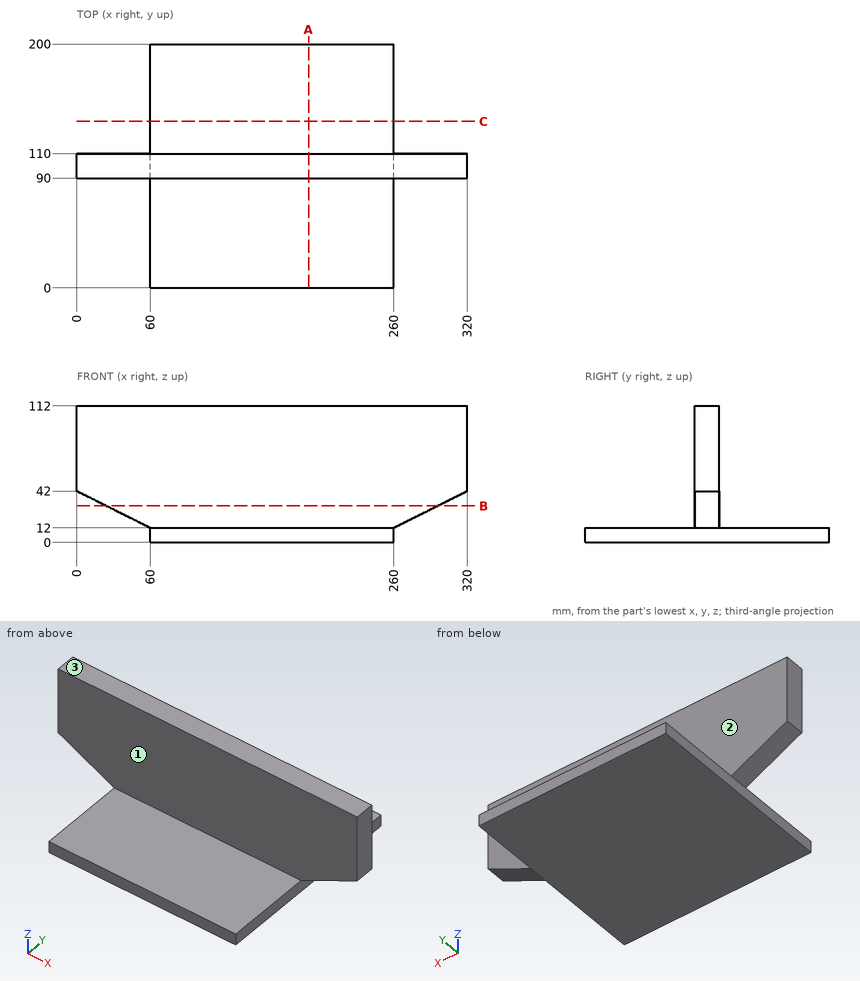
Input: dimensioned drawing with shaded views. Units: mm. Origin: part minimum x, y, z. A direction names the side the tool comes from. Round coordinates to 2 decimals unless told otherwise and drop trailing zeros. Loops run counter-clockwise (first coordinate to the right, second up) from the corner with the lowest first, then second, coordinate; pieces in that order, holes last. Notation, with made-up numbers: (-37.5, 49.5) -> (-4.5, 49.5) arc R16 ccw to (-4.5, 70.5) -> close; hole circle Ø1 at (60, 46). An arc over 180 degrees is marked (long way). Answer as a JSON object with one key per item and string values. Group by question number.
1) Ray query, L1, parallel to Y at x = 292.5, z = 94; L2, parallel to Z at x = 102.5, y = 60; L3, parallel to X at y = 32, z = 11. Return the intervals inside material, ascending.
2) Section query A-A on x = 190. Output: boundary loops of the cut face in (y, z).
3) Pin query (flat end, axial travel): pin 1 (1 mm diameter, centred on x = 113, z = 24.5, fed in from -Y); pin 2 (1 mm diameter, centred on x = 215.5, z = 25.5, fed in from +Y); pin 3 (6 mm diameter, centred on y = 82, z = 6.5, fed in from -X). Return the tip coordinate at first contact, or that it passes through.
4) Section query B-B on z = 30. Output: boundary loops of the cut face in (x, y).
5) Reachability of the marked faces 1, 2 and 3 from +Z, -Z, +X, -X, +Y, -Y: full face, straight path, thin tool, end or side. Return the list, or none.
6) Section query C-C on y = 136.5. Output: boundary loops of the cut face in (x, z), plus the area to 3 significant figures.
Reply:
{
 "1": {"L1": "y = 90 to 110", "L2": "z = 0 to 12", "L3": "x = 60 to 260"},
 "2": {"outline": "(0, 0) -> (200, 0) -> (200, 12) -> (110, 12) -> (110, 112) -> (90, 112) -> (90, 12) -> (0, 12) -> close"},
 "3": {"pin 1": "stops at y = 90", "pin 2": "stops at y = 110", "pin 3": "stops at x = 60"},
 "4": {"outline": "(24, 90) -> (296, 90) -> (296, 110) -> (24, 110) -> close"},
 "5": {"face 1": "+Z, +X, -X, -Y", "face 2": "+Z, +X, -X, +Y", "face 3": "+Z, +X, -X, +Y, -Y"},
 "6": {"outline": "(60, 0) -> (260, 0) -> (260, 12) -> (60, 12) -> close", "area": "2,400 mm2"}
}
